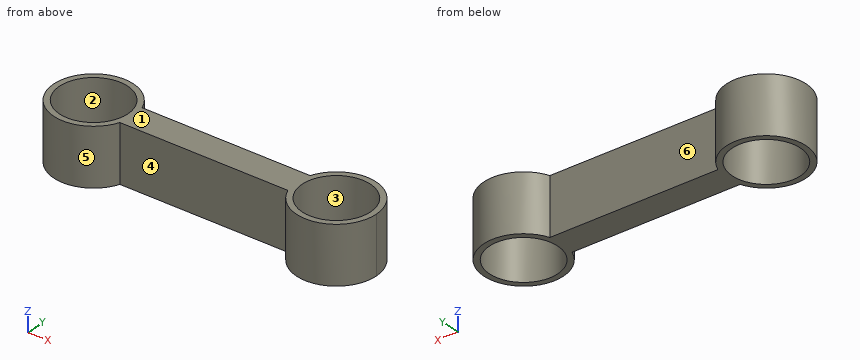
from build123d import *

# Parameters (mm, degrees)
SKETCH1_R           = 15.24
BOSS_EXTRUDE1_DEPTH = 25.4


with BuildPart() as part:
    # Sketch1 → Boss-Extrude1 (new body)
    with BuildSketch(Plane.XY):
        with BuildLine():
            ThreePointArc((16.607404975, 6.35), (-17.78, 0), (16.607404975, -6.35))
            Line((16.607404975, -6.35), (16.607404975, 6.35))
        make_face()
        Circle(SKETCH1_R, mode=Mode.SUBTRACT)
        with BuildLine():
            Line((16.607404975, -6.35), (91.342595025, -6.35))
            ThreePointArc((91.342595025, -6.35), (90.17, 0), (91.342595025, 6.35))
            Line((91.342595025, 6.35), (16.607404975, 6.35))
            ThreePointArc((16.607404975, 6.35), (17.484393905, 3.228679261), (17.78, 0))
            ThreePointArc((17.78, 0), (17.484393905, -3.228679261), (16.607404975, -6.35))
        make_face()
        with BuildLine():
            Line((16.607404975, 6.35), (16.607404975, -6.35))
            ThreePointArc((16.607404975, -6.35), (17.484393905, -3.228679261), (17.78, 0))
            ThreePointArc((17.78, 0), (17.484393905, 3.228679261), (16.607404975, 6.35))
        make_face()
        with BuildLine():
            Line((91.342595025, 6.35), (91.342595025, -6.35))
            ThreePointArc((91.342595025, -6.35), (111.178679261, -17.484393905), (125.73, 0))
            ThreePointArc((125.73, 0), (111.178679261, 17.484393905), (91.342595025, 6.35))
        make_face()
        with Locations((107.95, 0)):
            Circle(SKETCH1_R, mode=Mode.SUBTRACT)
        with BuildLine():
            ThreePointArc((91.342595025, 6.35), (90.17, 0), (91.342595025, -6.35))
            Line((91.342595025, -6.35), (91.342595025, 6.35))
        make_face()
    extrude(amount=BOSS_EXTRUDE1_DEPTH)


solid = part.part
Could you check a few things on this model? Use its own coordinates, in mm. Face numbers are marked on the shaded views. A direction names the side the tool comes from. Coordinates: 2 decimals unless noted, no trailing zeros. Write each loop counter-clockwise with the first axis right and the second up, starting at its lowest first coordinate (ties: lowest second). Pieces come first, ordered by that corner, then holes. Notation, with made-up numbers: (-35.75, 68.5) - (2.25, 68.5) arc R17 ccw to (2.25, 80.5) - close; hole circle Ø11 at (69, -36). An arc over 180 degrees is marked (long way). Put each result on its own line as item: value. Start each with the question number.
Q1. I want a section at A-A on z = 5. Write out the boundary of the cut face in (x, y), plus the area to 3 significant figures.
Q2. Thinking about a two-plate mould opening in X: for the marked faces 1, 2 and 3, which applies, pulls with the +X half, pulls with the -X half, needs draft (parallel to the pull), parting line crosses it, or undercut?
Q3. I want a section at C-C on y = -12.5. Write out the boundary of the cut face in (x, z), plus the area to 3 significant figures.
Q4. Please list where these lines run through material, in increasing order: L1, parallel to Y at x = 107.95, z = 6.5; L2, parallel to X at y = -9.5, z = 8; L3, parallel to X at y = -0.5, z = 24.
Q5. I want a section at D-D on y = -2. Write out the boundary of the cut face in (x, z), plus the area to 3 significant figures.
Q6. I want a section at B-B on x = 0. Write out the boundary of the cut face in (y, z).
Q7. I'm going to push flat-ended pins straight in: P1, Ø6, axis at y = -9, z = 10, coming from the +X side; P2, Ø12.5, axis at x = 54.5, z = 10, coming from the +Y side; P3, Ø12.5, axis at x = 72, z = 16, coming from the -Y side. Where does each tip first touch, or does it pass through?
Q8. Which directions (+Z, -Z, +X, -X, +Y, -Y) give clear straight access to the entire face, cutting with the end or side of a thin tool? Please do the marked faces 4, 5 and 6.
Checks:
1. outline: (16.61, -6.35) - (91.34, -6.35) arc R17.78 ccw (long way) to (91.34, 6.35) - (16.61, 6.35) arc R17.78 ccw (long way) to start; hole circle Ø30.48 at (0, 0); hole circle Ø30.48 at (107.95, 0)
1. area: 1,460 mm²
2. face 1: needs draft
2. face 2: undercut
2. face 3: undercut
3. outline: (-12.64, 0) - (-8.72, 0) - (-8.72, 25.4) - (-12.64, 25.4) - close; (8.72, 0) - (12.64, 0) - (12.64, 25.4) - (8.72, 25.4) - close; (95.31, 0) - (99.23, 0) - (99.23, 25.4) - (95.31, 25.4) - close; (116.67, 0) - (120.59, 0) - (120.59, 25.4) - (116.67, 25.4) - close
3. area: 399 mm²
4. L1: -17.78 to -15.24, 15.24 to 17.78
4. L2: -15.03 to -11.92, 11.92 to 15.03, 92.92 to 96.03, 119.87 to 122.98
4. L3: -17.77 to -15.23, 15.23 to 92.72, 123.18 to 125.72
5. outline: (-17.67, 0) - (-15.11, 0) - (-15.11, 25.4) - (-17.67, 25.4) - close; (15.11, 0) - (92.84, 0) - (92.84, 25.4) - (15.11, 25.4) - close; (123.06, 0) - (125.62, 0) - (125.62, 25.4) - (123.06, 25.4) - close
5. area: 2,100 mm²
6. outline: (-17.78, 0) - (-15.24, 0) - (-15.24, 25.4) - (-17.78, 25.4) - close; (15.24, 0) - (17.78, 0) - (17.78, 25.4) - (15.24, 25.4) - close
7. P1: x = 124.69
7. P2: y = 6.35
7. P3: y = -6.35
8. face 4: +Z, -Z, -Y
8. face 5: +Z, -Z
8. face 6: +Z, -Z, +Y
